from build123d import *

# Parameters (mm, degrees)
SKETCH2_R           = 21.0185
BOSS_EXTRUDE1_DEPTH = 71.12
SKETCH3_R           = 10.9855
BOSS_EXTRUDE2_DEPTH = 1.905
SKETCH4_R           = 10.9855
SKETCH4_R_2         = 8.4455
BOSS_EXTRUDE3_DEPTH = 1.905
SKETCH5_R           = 3
BOSS_EXTRUDE4_DEPTH = 25.4
SKETCH6_R           = 5.08
BOSS_EXTRUDE5_DEPTH = 3.429
SKETCH7_R           = 1.27
CUT_EXTRUDE1_DEPTH  = 5.08


with BuildPart() as part:
    # Sketch2 → Boss-Extrude1 (new body)
    with BuildSketch(Plane(origin=(0, 0, 0), x_dir=(1, 0, 0), z_dir=(0, 1, 0))):
        Circle(SKETCH2_R)
    extrude(amount=BOSS_EXTRUDE1_DEPTH)

    # Sketch3 → Boss-Extrude2 (add)
    with BuildSketch(Plane(origin=(0, 71.12, 0), x_dir=(1, 0, 0), z_dir=(0, 1, 0))):
        Circle(SKETCH3_R)
    extrude(amount=BOSS_EXTRUDE2_DEPTH)

    # Sketch4 → Boss-Extrude3 (add)
    with BuildSketch(Plane.XZ):
        Circle(SKETCH4_R)
        Circle(SKETCH4_R_2, mode=Mode.SUBTRACT)
    extrude(amount=BOSS_EXTRUDE3_DEPTH)

    # Sketch5 → Boss-Extrude4 (add)
    with BuildSketch(Plane.XZ):
        Circle(SKETCH5_R)
    extrude(amount=BOSS_EXTRUDE4_DEPTH)

    # Sketch6 → Boss-Extrude5 (add)
    with BuildSketch(Plane.XZ):
        Circle(SKETCH6_R)
    extrude(amount=BOSS_EXTRUDE5_DEPTH)

    # Sketch7 → Cut-Extrude1 (cut)
    with BuildSketch(Plane.XZ):
        with Locations((16, 0)):
            Circle(SKETCH7_R)
        with Locations((-16, 0)):
            Circle(SKETCH7_R)
    extrude(amount=-CUT_EXTRUDE1_DEPTH, mode=Mode.SUBTRACT)


solid = part.part
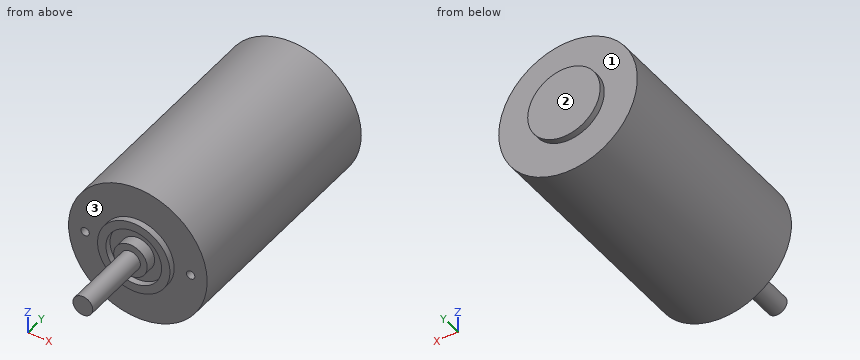
The model under review builds one solid part; all positions refer to its coordinate system, in mm. Face numbers are marked on the shaded views. A direction names the side the tool comes from. Give positions to 0.01 mm unless a question says otherwise; leave off trailing zeros. Write each loop counter-clockwise with the first axis right and the second up, starting at its lowest first coordinate (ties: lowest second). Pieces come first, ordered by that corner, then holes.
1. Add section A-A, the plane x = 0. Write out the cut boundary in (y, z) (1 decimal).
2. For P1, Ø4, axis at x = -17, y = -0.5, coming from the +Z side; P2, Ø1.3, axis at x = 16, z = -0.5, coming from the -Y side; P3, Ø3, axis at y = 27.5, z = 5, coming from the -X side; P4, Ø11, axis at x = -2, z = -4.5, coming from the -Y side, all flat-tipped, find the tip position at first contact; note any pin that passes through.
3. Add section D-D, the plane x = -16. Write out the cut boundary in (y, z).
4. Tool access review of the marked faces 1, 2 and 3: name each direction out of +Z, -Z, +X, -X, +Y, -Y from which nothing blocks a thin tool from reaching the whole face with its end or side.
5. Add section C-C, the plane y = -8. Write out the cut boundary in (x, z), plus the area to 3 significant figures.
6. Wall thickness on L1, parallel to Z at x = 0, y = -1.4; L2, parallel to Y at x = 2.5, z = -8.5 (3 decimals); L3, parallel to Y at x = -19, z = 8: over which ranges is each line inside the solid? List them lowest first.
Worked answers:
1. outline: (-25.4, -3) - (-3.4, -3) - (-3.4, -5.1) - (0, -5.1) - (0, -8.4) - (-1.9, -8.4) - (-1.9, -11) - (0, -11) - (0, -21) - (71.1, -21) - (71.1, -11) - (73, -11) - (73, 11) - (71.1, 11) - (71.1, 21) - (0, 21) - (0, 11) - (-1.9, 11) - (-1.9, 8.4) - (0, 8.4) - (0, 5.1) - (-3.4, 5.1) - (-3.4, 3) - (-25.4, 3) - close
2. P1: stops at z = 14.66
2. P2: stops at y = 5.08
2. P3: stops at x = -20.73
2. P4: stops at y = -25.4
3. outline: (0, -13.63) - (71.12, -13.63) - (71.12, 13.63) - (0, 13.63) - (0, 1.27) - (5.08, 1.27) - (5.08, -1.27) - (0, -1.27) - close
4. face 1: +Y
4. face 2: +Z, -Z, +X, -X, +Y
4. face 3: -Y
5. outline: circle Ø6 at (0, 0)
5. area: 28.3 mm2
6. L1: z = -10.99 to -8.45, -5.08 to 5.08, 8.45 to 10.99
6. L2: y = -1.905 to 73.025
6. L3: y = 0 to 71.12
